```python
from build123d import *

# Parameters (mm, degrees)
BOSS_EXTRUDE1_DEPTH = 98
SKETCH2_R           = 2.5
CUT_EXTRUDE1_DEPTH  = 8


with BuildPart() as part:
    # Sketch1 → Boss-Extrude1 (new body, symmetric)
    with BuildSketch(Plane.XY):
        Polygon((-2.585786438, 4), (2.585786438, 4), (6.585786438, 8), (2.5, 8), (2.5, 10), (10, 10), (10, 2.5), (8, 2.5), (8, 6.585786438), (4, 2.585786438), (4, -2.585786438), (8, -6.585786438), (8, -2.5), (10, -2.5), (10, -10), (2.5, -10), (2.5, -8), (6.585786438, -8), (2.585786438, -4), (-2.585786438, -4), (-6.585786438, -8), (-2.5, -8), (-2.5, -10), (-10, -10), (-10, -2.5), (-8, -2.5), (-8, -6.585786438), (-4, -2.585786438), (-4, 2.585786438), (-8, 6.585786438), (-8, 2.5), (-10, 2.5), (-10, 10), (-2.5, 10), (-2.5, 8), (-6.585786438, 8), align=None)
    extrude(amount=BOSS_EXTRUDE1_DEPTH, both=True)

    # Sketch2 → Cut-Extrude1 (cut)
    with BuildSketch(Plane(origin=(4, 0, 0), x_dir=(0, 0, -1), z_dir=(1, 0, 0))):
        with Locations((88, 0)):
            Circle(SKETCH2_R)
        with Locations((-88, 0)):
            Circle(SKETCH2_R)
    extrude(amount=-CUT_EXTRUDE1_DEPTH, mode=Mode.SUBTRACT)


solid = part.part
```
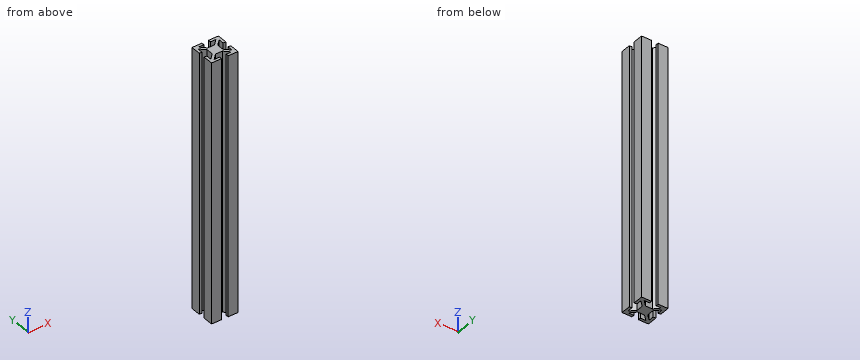
Model file for the job. Use its own axes, mm. Coordinates: 2 decimals unless noted, no trailing zeros. Order: outer loops, then holes, each group sorted by start corner. A loop starts at its lowest first (then second) coordinate and runs counter-clockwise, first axis right, second up. Notation, with made-up numbers: M 20,66.25 L 78,66.25 A26 ccw 78,87.25 Z; hole C -7.75,69.5 d4. An arc over 180 degrees is marked long. Answer as CSV lines item,"result".
(1) Flat gauge pin, fed straight in: pin 1 (4.5 mm diameter, centred on y = 0, z = 88, fed in from -X). Where does the tip first touch, or does it go through?
Geometry says:
pin 1,"passes through"
(2) Wall check: line 1 along Y through (x, z) = (-8.25, 38.5); line 2 along X through (y, z) = (4.25, 78.5); line 3 along Y through (x, z) = (1, -88). Give the ranges that are in metal, low to high.
Geometry says:
line 1,"y = -10 to -2.5, 2.5 to 10"
line 2,"x = -10 to -8, -5.66 to -2.84, 2.84 to 5.66, 8 to 10"
line 3,"y = -4 to -2.5, 2.5 to 4"
(3) Band-saw the part on A-A, the plane y = 0. List the corners of the cut face in (x, z).
Geometry says:
outline,"M -4,-98 L 4,-98 L 4,-90.5 L -4,-90.5 Z; M -4,-85.5 L 4,-85.5 L 4,85.5 L -4,85.5 Z; M -4,90.5 L 4,90.5 L 4,98 L -4,98 Z"
(4) Band-saw the part on B-B, the plane x = 0.5. List the corners of the cut face in (y, z).
Geometry says:
outline,"M -4,-98 L 4,-98 L 4,98 L -4,98 Z; hole C 0,-88 d5; hole C 0,88 d5"
